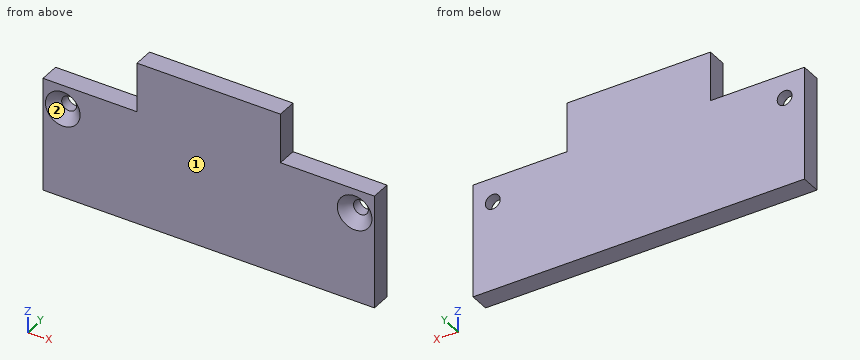
Autodesk Inventor part; units mm, degrees
ref_plane "YZ Plane" through (0, 0, 0) normal (1, 0, 0) x (0, 1, 0)
ref_plane "XZ Plane" through (0, 0, 0) normal (0, 1, 0) x (-1, 0, 0)
ref_plane "XY Plane" through (0, 0, 0) normal (0, 0, 1) x (1, 0, 0)
sketch "Sketch1" plane through (0, 0, 0) normal (0, 1, 0) x (-1, 0, 0)
  line L0 (-33.5, -11.5) -> (33.5, -11.5)
  line L1 (33.5, -11.5) -> (33.5, 11.5)
  line L2 (33.5, 11.5) -> (-33.5, 11.5)
  line L3 (-33.5, 11.5) -> (-33.5, -11.5)
  line L4 (-33.5, -11.5) -> (33.5, 11.5) construction
  line L5 (33.5, -11.5) -> (-33.5, 11.5) construction
  line L6 (-14.5, 21.5) -> (14.5, 21.5)
  line L7 (14.5, 21.5) -> (14.5, 11.5)
  line L8 (14.5, 11.5) -> (-14.5, 11.5)
  line L9 (-14.5, 11.5) -> (-14.5, 21.5)
  line L10 (-14.5, 21.5) -> (14.5, 11.5) construction
  line L11 (14.5, 21.5) -> (-14.5, 11.5) construction
  point P0 (0, 0)
  point P1 (0, 16.5)
  point P2 (0, 0)
  point P3 (0, 16.5)
  point P4 (-14.5, 11.5)
  dimension "d0" = 67
  dimension "d1" = 23
  dimension "d2" = 29
  dimension "d3" = 10
extrude "Extrusion1" add sketch "Sketch1" along normal blind 4
sketch "Sketch2" plane through (0, 4, 0) normal (0, 1, 0) x (1, 0, 0)
  circle A0 centre (-29.5, -6.625) radius 1.5
  circle A1 centre (29.5, -6.625) radius 1.5
  line L0 (33.5, -11.5) -> (33.5, 11.5)
  line L1 (-33.5, 11.5) -> (-33.5, -11.5)
  line L2 (33.5, 11.5) -> (-33.5, 11.5)
  point P0 (0, 0)
  dimension "d6" = 4
  dimension "d7" = 4
  dimension "d8" = 18.125
  dimension "d9" = 18.125
  dimension "d10" = 3
extrude "Extrusion2" cut sketch "Sketch2" against normal through all
chamfer "Chamfer1" distance 2 angle 45 2 edges at (28, 0, 6.625) (-31, 0, 6.625)
equation "\"d7\" = d6"
equation "\"d9\" = d8"
properties part number "WeightFront" material "Lead"
For this review, take the finished solid that the model builds, in its own axes (mm). Face numbers are marked on the shaded views. Round coordinates to 2 decimals unless told otherwise and drop trailing zeros. Order: outer loops, then holes, each group sorted by start corner. A loop starts at its lowest first (then second) coordinate and runs counter-clockwise, first axis right, second up. Notation, with made-up numbers: (41, 57) -> (49, 57) arc R26 ccw to (49, 81) -> close; hole circle Ø7 at (58, 24). An arc over 180 degrees is marked (long way). Use a Markdown table: item, result.
Item 1: Take a section at B-B (y = 0.85). State the section outline as (x, z) points (3 decimals), plus the area to 3 significant figures.
Resolved:
| item | result |
|---|---|
| outline | (-33.5, -11.5) -> (33.5, -11.5) -> (33.5, 11.5) -> (14.5, 11.5) -> (14.5, 21.5) -> (-14.5, 21.5) -> (-14.5, 11.5) -> (-33.5, 11.5) -> close; hole circle Ø5.3 at (-29.5, 6.625); hole circle Ø5.3 at (29.5, 6.625) |
| area | 1,790 mm² |
Item 2: For pin 1 (2.5 mm diameter, centred on x = 29.5, z = 6.625, fed in from +Y); pin 2 (6 mm diameter, centred on x = -6, z = 3.5, fed in from -Y); pin 3 (1.2 mm diameter, centred on y = 2.5, z = 18.5, fed in from +X); pin 4 (1.2 mm diameter, centred on x = 23, y = 2, fed in from +Z), all flat-tipped, find the tip position at first contact; note any pin that passes through.
Resolved:
| item | result |
|---|---|
| pin 1 | passes through |
| pin 2 | stops at y = 0 |
| pin 3 | stops at x = 14.5 |
| pin 4 | stops at z = 11.5 |
Item 3: Take a section at A-A (x = -29.5). State the section outline as (y, z) points (3 decimals).
Resolved:
| item | result |
|---|---|
| outline | (0, -11.5) -> (4, -11.5) -> (4, 5.125) -> (2, 5.125) -> (0, 3.125) -> close; (0, 10.125) -> (2, 8.125) -> (4, 8.125) -> (4, 11.5) -> (0, 11.5) -> close |
Item 4: Take a section at C-C (z = 15.5). State the section outline as (x, y) points.
Resolved:
| item | result |
|---|---|
| outline | (-14.5, 0) -> (14.5, 0) -> (14.5, 4) -> (-14.5, 4) -> close |
Item 5: Draft analysis for pull direction X (two halves, no side actions). For the marked faces 1 and 2, state which applies: +X half, -X half, draft (parallel to the pull), parting line (faces both ways), or undercut.
Resolved:
| item | result |
|---|---|
| face 1 | draft |
| face 2 | undercut |
Item 6: For line 1 along Z through (x, y) = (-29.5, 3.15) (3 decimals); line 2 along X through (y, z) = (3.7, 6); line 3 along X through (y, z) = (1.15, 7.5), list the stretches that pass through material, from the lowest coordinate up. Write a range as [from, to].
Resolved:
| item | result |
|---|---|
| line 1 | z = [-11.5, 5.125], [8.125, 11.5] |
| line 2 | x = [-33.5, -30.86], [-28.14, 28.14], [30.86, 33.5] |
| line 3 | x = [-33.5, -31.68], [-27.32, 27.32], [31.68, 33.5] |
Item 7: Take a section at D-D (x = -16.5). State the section outline as (y, z) points.
Resolved:
| item | result |
|---|---|
| outline | (0, -11.5) -> (4, -11.5) -> (4, 11.5) -> (0, 11.5) -> close |
